Check sheet for the modelled part. Datum: model origin and axes. Units: mm. A direction names the side the tool comes from. Coordinates: 2 decimals unless noted, no trailing zeros. Loops run counter-clockwise (first coordinate to the right, second up) from the corner with the lowest first, then second, coordinate; pieces in that order, holes last. Notation, with made-up numbers: (61.5, 26) - (120.5, 26) arc R24 ccw to (120.5, 53) - close; hole circle Ø3 at (-13, 16.5). An arc over 180 degrees is marked (long way). Write each question's results on one line, items separated by ' | '. Start each with the question number.
1. Cross-section at D-D (x = -11). Record the cut outline in (y, z).
2. Gauge pin test, flat ends, axial feed: P1, Ø1.5, axis at x = 7.75, z = -13.42, coming from the +Y side; P2, Ø3, axis at x = -7.75, z = -13.42, coming from the +Y side; P3, Ø8, axis at y = -7.5, z = 7, coming from the -X side. Record the tip position at first contact, or that the pin passes through.
3. Cross-section at C-C (y = 34.5). Record the cut outline in (x, z).
4. Cross-section at A-A (x = 10). Record the cut outline in (y, z), and give its area (3 significant figures).
5. Cross-section at B-B (z = -7). Record the cut outline in (x, y).
6. Tool access check on faces 5 (the face through (8.26, -10.85, -15.88)), 6 (the face through (0, 42, -9.5)), 7 (the face through (14.31, 23.23, -0.38)), 8 (the face through (0, -22, 0)), 9 (the face through (0, 46.5, -7)). Record the directions out of +Z, -Z, +X, -X, +Y, -Y that give a thin tool (end or side, any length) a straight path to the whole face; none if there is none.
7. Thickness scan on line 1 (Z direction, x = 7.75, y = 23.95); line 2 (Z direction, x = -7, y = 23); line 3 (Y direction, x = 8.5, z = 9). Record the ranges inside material, lowest first. Write a range as [from, to].
8. Draft check along Z on faces 1 (the face through (-15.3, 20.88, 0.08)), 2 (the face through (-0.78, 27.96, -12.95)), 3 (the face through (-8, 20.9, 13.4)), 4 (the face through (-3, 31, -6)). Enter one of: released by +Z, released by -Z, zero draft, split by the parting line, or undercut.
```python
from build123d import *

# Parameters (mm, degrees)
SKETCH1_R                       = 18.499999957
BOSS_EXTRUDE1_DEPTH             = 25.000000038
SKETCH2_R                       = 5.999999938
BOSS_EXTRUDE2_DEPTH             = 5.999999938
BOSS_EXTRUDE3_DEPTH             = 15.499999988
BOSS_EXTRUDE4_DEPTH             = 5.999999938
TAP_DRILL_FOR_M3X0_5_TAP1_D     = 2.5
TAP_DRILL_FOR_M3X0_5_TAP1_DEPTH = 3.499993
TAP_DRILL_FOR_M3X0_5_TAP1_TIP   = 0.751075774
SKETCH7_R                       = 17.900000014
BOSS_EXTRUDE5_DEPTH             = 21.999999942


with BuildPart() as part:
    # Sketch1 → Boss-Extrude1 (new body)
    with BuildSketch(Plane(origin=(0, 0, 0), x_dir=(1, 0, 0), z_dir=(0, 1, 0))):
        Circle(SKETCH1_R)
    extrude(amount=BOSS_EXTRUDE1_DEPTH)

    # Sketch2 → Boss-Extrude2 (add)
    with BuildSketch(Plane(origin=(0, 25.000000038, 0), x_dir=(1, 0, 0), z_dir=(0, 1, 0))):
        with Locations((0, 6.99999997)):
            Circle(SKETCH2_R)
    extrude(amount=BOSS_EXTRUDE2_DEPTH)

    # Sketch3 → Boss-Extrude3 (add)
    with BuildSketch(Plane(origin=(0, 30.999999976, 0), x_dir=(1, 0, 0), z_dir=(0, 1, 0))):
        with BuildLine():
            Line((-1.658312218, 9.50000005), (1.658312218, 9.50000005))
            ThreePointArc((1.658312218, 9.50000005), (0, 4.000000001), (-1.658312218, 9.50000005))
        make_face()
    extrude(amount=BOSS_EXTRUDE3_DEPTH)

    # Sketch3_3 → Boss-Extrude4 (add)
    with BuildSketch(Plane(origin=(0, 30.999999976, 0), x_dir=(1, 0, 0), z_dir=(0, 1, 0))):
        with BuildLine():
            Line((-1.658312218, 9.50000005), (1.658312218, 9.50000005))
            ThreePointArc((1.658312218, 9.50000005), (0, 9.999999939), (-1.658312218, 9.50000005))
        make_face()
    extrude(amount=BOSS_EXTRUDE4_DEPTH)

    # Tap Drill for M3x0.5 Tap1
    with Locations(Plane(origin=(0, 25.000000038, 0), x_dir=(1, 0, 0), z_dir=(0, 1, 0))):
        with Locations((-15.499999988, 0), (-7.749999994, 13.423393748), (7.749999994, 13.423393748), (15.499999988, 0), (7.749999994, -13.423393748), (-7.749999994, -13.423393748)):
            Hole(TAP_DRILL_FOR_M3X0_5_TAP1_D / 2, depth=TAP_DRILL_FOR_M3X0_5_TAP1_DEPTH)
            with Locations((0, 0, -(TAP_DRILL_FOR_M3X0_5_TAP1_DEPTH + TAP_DRILL_FOR_M3X0_5_TAP1_TIP / 2))):  # 118° drill point
                Cone(0, TAP_DRILL_FOR_M3X0_5_TAP1_D / 2, TAP_DRILL_FOR_M3X0_5_TAP1_TIP, mode=Mode.SUBTRACT)

    # Sketch7 → Boss-Extrude5 (add)
    with BuildSketch(Plane.XZ):
        Circle(SKETCH7_R)
    extrude(amount=BOSS_EXTRUDE5_DEPTH)


solid = part.part
```
Established:
1) outline: (-22, -14.12) - (0, -14.12) - (0, -14.87) - (25, -14.87) - (25, 14.87) - (0, 14.87) - (0, 14.12) - (-22, 14.12) - close
2) P1: y = 21.2 | P2: y = 25 | P3: x = -17.65
3) outline: circle Ø6 at (0, -7)
4) outline: (-22, -14.85) - (0, -14.85) - (0, -15.56) - (25, -15.56) - (25, 15.56) - (0, 15.56) - (0, 14.85) - (-22, 14.85) - close | area: 1,430 mm^2
5) outline: (-17.12, 0) - (-16.47, 0) - (-16.47, -22) - (16.47, -22) - (16.47, 0) - (17.12, 0) - (17.12, 25) - (6, 25) - (6, 31) - (3, 31) - (3, 46.5) - (-3, 46.5) - (-3, 31) - (-6, 31) - (-6, 25) - (-17.12, 25) - close
6) face 5: -Y | face 6: -Z, +X, -X, +Y | face 7: +Y | face 8: +Z, -Z, +X, -X, -Y | face 9: +Z, -Z, +X, -X, +Y
7) line 1: [-16.8, -14.67], [-12.17, 12.17], [14.67, 16.8] | line 2: [-17.12, -14.42], [-12.42, 12.42], [14.42, 17.12] | line 3: [-22, 25]
8) face 1: undercut | face 2: split by the parting line | face 3: undercut | face 4: zero draft
